from build123d import *

# Parameters (mm, degrees)
SKETCH1_R           = 2.75
BOSS_EXTRUDE1_DEPTH = 5
BOSS_EXTRUDE2_DEPTH = 5
RADYUS2_R           = 0.5
RADYUS3_R           = 1
RADYUS4_R           = 1
SKETCH3_R           = 1.5
CUT_EXTRUDE1_DEPTH  = 34.719430671
RADYUS5_R           = 1


with BuildPart() as part:
    # Sketch1 → Boss-Extrude1 (new body)
    with BuildSketch(Plane(origin=(0, 0, 0), x_dir=(1, 0, 0), z_dir=(0, 1, 0))):
        with BuildLine():
            Line((-21.5, 2.5), (-21.5, -2.5))
            Line((-21.5, -2.5), (-3.564762336, -9.343043909))
            ThreePointArc((-3.564762336, -9.343043909), (0, -10), (3.564762336, -9.343043909))
            Line((3.564762336, -9.343043909), (21.5, -2.5))
            Line((21.5, -2.5), (21.5, 2.5))
            Line((21.5, 2.5), (7.5, 7.841586018))
            Line((7.5, 7.841586018), (7.5, 14))
            Line((7.5, 14), (0.5, 14))
            Line((0.5, 14), (0.5, 9.987492178))
            Line((0.5, 9.987492178), (0.5, 3.968626967))
            ThreePointArc((0.5, 3.968626967), (0, -4), (-0.5, 3.968626967))
            Line((-0.5, 3.968626967), (-0.5, 9.987492178))
            Line((-0.5, 9.987492178), (-0.5, 14))
            Line((-0.5, 14), (-7.5, 14))
            Line((-7.5, 14), (-7.5, 7.841586018))
            Line((-7.5, 7.841586018), (-21.5, 2.5))
        make_face()
        with Locations(Location((-16, 0, 0), (0, 0, 270))):
            Circle(SKETCH1_R, mode=Mode.SUBTRACT)
        with Locations(Location((16, 0, 0), (0, 0, 270))):
            Circle(SKETCH1_R, mode=Mode.SUBTRACT)
    extrude(amount=BOSS_EXTRUDE1_DEPTH)

    # Sketch2 → Boss-Extrude2 (add)
    with BuildSketch(Plane(origin=(0, 5, 0), x_dir=(1, 0, 0), z_dir=(0, 1, 0))):
        with BuildLine():
            Line((-0.5, 3.968626967), (-0.5, 9.987492178))
            ThreePointArc((-0.5, 9.987492178), (0, -10), (0.5, 9.987492178))
            Line((0.5, 9.987492178), (0.5, 3.968626967))
            ThreePointArc((0.5, 3.968626967), (0, -4), (-0.5, 3.968626967))
        make_face()
    extrude(amount=BOSS_EXTRUDE2_DEPTH)

    # Radyus2
    radyus2_edges = [part.edges().sort_by_distance(p)[0] for p in [
        (0, 10, 10),
    ]]
    fillet(radyus2_edges, radius=RADYUS2_R)

    # Radyus3
    radyus3_edges = [part.edges().sort_by_distance(p)[0] for p in [
        (21.5, 2.5, 2.5),
    ]]
    fillet(radyus3_edges, radius=RADYUS3_R)

    # Radyus4
    radyus4_edges = [part.edges().sort_by_distance(p)[0] for p in [
        (-21.5, 2.5, -2.5),
        (-21.5, 2.5, 2.5),
        (21.5, 2.5, -2.5),
    ]]
    fillet(radyus4_edges, radius=RADYUS4_R)

    # Sketch3 → Cut-Extrude1 (cut, through all)
    with BuildSketch(Plane(origin=(7.5, 0, 0), x_dir=(0, 0, -1), z_dir=(1, 0, 0))):
        with Locations((10.920793009, 2.5)):
            Circle(SKETCH3_R)
    extrude(amount=-CUT_EXTRUDE1_DEPTH, mode=Mode.SUBTRACT)

    # Radyus5
    radyus5_edges = [part.edges().sort_by_distance(p)[0] for p in [
        (7.5, 2.5, -14),
        (-7.5, 2.5, -14),
    ]]
    fillet(radyus5_edges, radius=RADYUS5_R)


solid = part.part
Model file for the job. Use its own axes, mm. A direction names the side the tool comes from. Give positions to 0.01 mm unless a question says otherwise; leave off trailing zeros. Loops run counter-clockwise (first coordinate to the right, second up) from the corner with the lowest first, then second, coordinate; pieces in that order, holes last.
Item 1: Which spindle directions (+Z, -Z, +X, -X, +Y, -Y) get a long thin tool onto all of the face, cutting with end or side? Do faces 5 (the face through (2, 10, 4)), 6 (the face through (-7.5, 2, -9)), 7 (the face through (0.5, 5, -8)), 8 (the face through (7.5, 2, -9)). Say none if no direction does.
Check values:
face 5: +Z, -Z, +X, -X, +Y
face 6: -Z, -X, +Y, -Y
face 7: -Z, +Y, -Y
face 8: -Z, +X, +Y, -Y
Item 2: Drop flat-ended pins along their axis: P1, Ø5, axis at y = 2.5, z = -10.92, coming from the -X side; P2, Ø3, axis at y = 7.5, z = -6.5, coming from the -X side; P3, Ø1.5, axis at y = 3, z = -10.5, coming from the -X side; P4, Ø4, axis at y = 4, z = 4.5, coming from the -X side (3 decimals). Give the stop position or say it passes through.
Check values:
P1: stops at x = -7.5
P2: stops at x = -8.66
P3: passes through
P4: stops at x = -21.225
Item 3: Drill centre lines: line 1 along X through (y, z) = (0.5, -10.25); line 2 along X through (y, z) = (1.2, 0); line 3 along Z through (x, y) = (1, 3.75). Where is each one in solid material? Low to high.
Check values:
line 1: x = -7.5 to -0.5, 0.5 to 7.5
line 2: x = -21.5 to -18.75, -13.25 to -4, 4 to 13.25, 18.75 to 21.5
line 3: z = -14 to -11.75, -10.09 to -3.87, 3.87 to 9.95
Item 4: Mould opens along Z. For faces 1 (the face through (-13.273, 2.465, -0.358)), 2 (the face through (0, 5, 4)), 3 (the face through (4.5, 0, 0.5)), 4 (the face through (-21.319, 2.535, 2.385)) say: +Z half, -Z half, draft (parallel to the pull), parting line (faces both ways), or undercut.
Check values:
face 1: undercut
face 2: undercut
face 3: draft
face 4: +Z half
Item 5: Slice it at C-C (x = 11.5). Write the cut outline in (y, z), plus the area to 3 significant figures.
Check values:
outline: (0, -6.32) - (5, -6.32) - (5, 6.32) - (0, 6.32) - close
area: 63.2 mm2
Item 6: Slice it at B-B (z = 0). Give the number of separate pieces and of enclosed holes in the cut face, plus the area to 3 significant figures.
Check values:
separate pieces: 4
enclosed holes: 0
area: 180 mm2
Item 7: Slice it at A-A (x = 16). Write the cut outline in (y, z), plus the area to 3 significant figures.
Check values:
outline: (0, -4.6) - (5, -4.6) - (5, -2.75) - (0, -2.75) - close; (0, 2.75) - (5, 2.75) - (5, 4.6) - (0, 4.6) - close
area: 18.5 mm2
